from build123d import *

# Parameters (mm, degrees)
ESBO_O2_W                                   = 15.5
ESBO_O2_H                                   = 30
RESSALTO_EXTRUS_O1_DEPTH                    = 15.5
ESBO_O3_R                                   = 1.5
RESSALTO_EXTRUS_O2_DEPTH                    = 7
ESBO_O4_R                                   = 2.75
RESSALTO_EXTRUS_O3_DEPTH                    = 23
BROCA_DE_ROSQUEAR_PARA_TARRAXA_DE_M31_D     = 2.5
BROCA_DE_ROSQUEAR_PARA_TARRAXA_DE_M31_DEPTH = 1.1
BROCA_DE_ROSQUEAR_PARA_TARRAXA_DE_M31_TIP   = 0.751075774


with BuildPart() as part:
    # Esboço2 → Ressalto-extrusão1 (new body)
    with BuildSketch(Plane.XY):
        with Locations((6.870290308, 0.804951604)):
            Rectangle(ESBO_O2_W, ESBO_O2_H)
    extrude(amount=RESSALTO_EXTRUS_O1_DEPTH)

    # Esboço3 → Ressalto-extrusão2 (add)
    with BuildSketch(Plane(origin=(0, 15.804951604, 0), x_dir=(1, 0, 0), z_dir=(0, 1, 0))):
        with Locations(Location((6.870290308, -7.75, 0), (0, 0, 90))):
            Circle(ESBO_O3_R)
    extrude(amount=RESSALTO_EXTRUS_O2_DEPTH)

    # Esboço4 → Ressalto-extrusão3 (add)
    with BuildSketch(Plane.XZ.offset(14.195048396)):
        with Locations(Location((6.870290308, 7.75, 0), (0, 0, 180))):
            Circle(ESBO_O4_R)
    extrude(amount=RESSALTO_EXTRUS_O3_DEPTH)

    # Broca de rosquear para tarraxa de M31
    with Locations(Plane(origin=(-0.879709692, 8.304951604, 7.75), x_dir=(0, -1, 0), z_dir=(-1, 0, 0))):
        with Locations((0, 0), (15, 0)):
            Hole(BROCA_DE_ROSQUEAR_PARA_TARRAXA_DE_M31_D / 2, depth=BROCA_DE_ROSQUEAR_PARA_TARRAXA_DE_M31_DEPTH)
            with Locations((0, 0, -(BROCA_DE_ROSQUEAR_PARA_TARRAXA_DE_M31_DEPTH + BROCA_DE_ROSQUEAR_PARA_TARRAXA_DE_M31_TIP / 2))):  # 118° drill point
                Cone(0, BROCA_DE_ROSQUEAR_PARA_TARRAXA_DE_M31_D / 2, BROCA_DE_ROSQUEAR_PARA_TARRAXA_DE_M31_TIP, mode=Mode.SUBTRACT)


solid = part.part
Here's how the part is built. I have some questions about the finished solid (model axes, mm). A direction names the side the tool comes from. Give positions to 0.01 mm unless a question says otherwise; leave off trailing zeros. Order: outer loops, then holes, each group sorted by start corner. A loop starts at its lowest first (then second) coordinate and runs counter-clockwise, first axis right, second up. Notation, with made-up numbers: (-32.5, -16) -> (23.5, -16) arc R13 ccw to (23.5, -5) -> close; hole circle Ø7 at (-10, 69.25). An arc over 180 degrees is marked (long way). One line per item, written item: value. Start each with the question number.
1. For faces 4 (the face through (7, -37.195, 8)), 5 (the face through (10, -14.195, 8)), 6 (the face through (6.8, 19.26, 9.25)), 7 (the face through (-0.322, -7.944, 7.805)), which set-ups out of +Z, -Z, +X, -X, +Y, -Y let a thin tool reach every point of the face, with its end or its side?
2. Imagine slicing it at B-B, the plane x = 9. List the corners of the cut face in (y, z) for me.
3. Will these pins go through, and if not, where does the flat tip stop? pin 1 Ø1.5 at (x, y) = (4, -12) entering from -Z; pin 2 Ø6 at (x, z) = (6, 12.5) entering from +Y; pin 3 Ø1.5 at (x, z) = (8.5, 4.5) entering from -Y.
4. Imagine slicing it at D-D, the plane y = 17. List the corners of the cut face in (x, z) for me.
5. I need wall thicknesses on probe 1 along Y at (x, z) = (-0.05, 7.75); probe 2 along Y at (x, z) = (3, 7); probe 3 along X at (y, z) = (-26.5, 7.5). Which ranges of each line are inside material? Lowest first, please. Write a range as from..to.
6. Imagine slicing it at A-A, the plane y = -30.5. List the corners of the cut face in (x, z) for me.
7. We'd pull the mould along Z, two halves only. Please class faces 1 (the face through (4.33, -25.53, 8.8)), 2 (the face through (-0.88, 1, 8)), 3 (the face through (0.84, 8.46, 7.9)): released by +Z, released by -Z, zero draft, split by the parting line, or undercut.
8. Imagine slicing it at C-C, the plane z = 14.75. List the corners of the cut face in (x, y) for me, plus the area to 3 significant figures.
Values follow:
1. face 4: +Z, -Z, +X, -X, -Y
1. face 5: -Y
1. face 6: +Y
1. face 7: -X
2. outline: (-37.2, 6.01) -> (-14.2, 6.01) -> (-14.2, 0) -> (15.8, 0) -> (15.8, 15.5) -> (-14.2, 15.5) -> (-14.2, 9.49) -> (-37.2, 9.49) -> close
3. pin 1: stops at z = 0
3. pin 2: stops at y = 15.8
3. pin 3: stops at y = -14.2
4. outline: circle Ø3 at (6.87, 7.75)
5. probe 1: y = -14.2..-7.95, -5.45..7.05, 9.55..15.8
5. probe 2: y = -14.2..15.8
5. probe 3: x = 4.13..9.61
6. outline: circle Ø5.5 at (6.87, 7.75)
7. face 1: split by the parting line
7. face 2: zero draft
7. face 3: undercut
8. outline: (-0.88, -14.2) -> (14.62, -14.2) -> (14.62, 15.8) -> (-0.88, 15.8) -> close
8. area: 465 mm2
